```python
from build123d import *

# Parameters (mm, degrees)
F0_R     = 57.5
F1_DEPTH = 18
F2_R     = 50
F3_DEPTH = 5
F5_DEPTH = 8


with BuildPart() as f1:
    # F0 (on Top) → F1 (new body)
    with BuildSketch(Plane.XY):
        Circle(F0_R)
    extrude(amount=F1_DEPTH)

    # F2 (on face) → F3 (cut)
    with BuildSketch(Plane(origin=(0, 0, 0), x_dir=(1, 0, 0), z_dir=(0, 0, -1))):
        Circle(F2_R)
    extrude(amount=-F3_DEPTH, mode=Mode.SUBTRACT)

    # F4 (on face) → F5 (cut)
    with BuildSketch(Plane(origin=(0, 0, 5), x_dir=(1, 0, 0), z_dir=(0, 0, -1))):
        with BuildLine():
            ThreePointArc((-2.8, 1.65), (-0.855132, -3.135482), (3.25, 0))
            ThreePointArc((3.25, 0), (3.135482, 0.855132), (2.8, 1.65))
            Line((2.8, 1.65), (-2.8, 1.65))
        make_face()
    extrude(amount=-F5_DEPTH, mode=Mode.SUBTRACT)


solid = f1.part
```
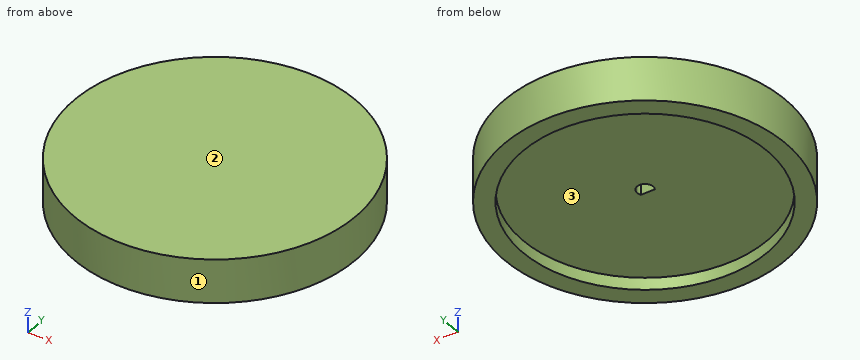
The model under review builds one solid part; all positions refer to its coordinate system, in mm. Face numbers are marked on the shaded views. Round coordinates to 2 decimals unless told otherwise and drop trailing zeros. Order: outer loops, then holes, each group sorted by start corner. A loop starts at its lowest first (then second) coordinate and runs counter-clockwise, first axis right, second up.
Item 1: Add section D-D, the plane z = 2. State the section outline as (x, y) points, and give its area (3 significant figures).
Working result:
outline: circle Ø115 at (0, 0); hole circle Ø100 at (0, 0)
area: 2,530 mm2
Item 2: To check wall thickness, follow probe 1 along Y at (x, z) = (0, 3.95); probe 2 along Y at (x, z) = (0, 10.5); probe 3 along Z at (x, y) = (-16.5, -13). State the ranges of each line that lie inside material, in increasing order.
Working result:
probe 1: y = -57.5 to -50, 50 to 57.5
probe 2: y = -57.5 to -1.65, 3.25 to 57.5
probe 3: z = 5 to 18
Item 3: Add section C-C, the plane z = 15.25. State the section outline as (x, y) points, and give its area (3 significant figures).
Working result:
outline: circle Ø115 at (0, 0)
area: 10,400 mm2
Item 4: For pin 1 (6 mm diameter, centred on x = 4.5, z = 13, fed in from -Y); pin 2 (5.5 mm diameter, centred on x = 0.5, y = 0.5, fed in from -Z); pin 3 (10 mm diameter, centred on x = -39.5, z = 12, fed in from +Y), all flat-tipped, find the tip position at first contact; note any pin that passes through.
Working result:
pin 1: stops at y = -57.48
pin 2: stops at z = 5
pin 3: stops at y = 46
Item 5: Add section A-A, the plane x = 0. State the section outline as (y, z) points.
Working result:
outline: (-57.5, 0) - (-50, 0) - (-50, 5) - (-1.65, 5) - (-1.65, 13) - (3.25, 13) - (3.25, 5) - (50, 5) - (50, 0) - (57.5, 0) - (57.5, 18) - (-57.5, 18) - close
Item 6: Draft analysis for pull direction Y (two halves, no side actions). For the marked faces 1, 2 and 3, state which applies: released by +Y, released by -Y, zero draft, split by the parting line, or undercut.
Working result:
face 1: split by the parting line
face 2: zero draft
face 3: undercut
Item 7: Add section B-B, the plane y = 22.5. State the section outline as (x, z) points.
Working result:
outline: (-52.92, 0) - (-44.65, 0) - (-44.65, 5) - (44.65, 5) - (44.65, 0) - (52.92, 0) - (52.92, 18) - (-52.92, 18) - close
